```python
from build123d import *

# Parameters (mm, degrees)
BOSS_EXTRUDE1_DEPTH   = 3
BOSS_EXTRUDE2_DEPTH   = 3.5
BOSS_EXTRUDE3_DEPTH   = 3.7
SKETCH4_R             = 2.88
BOSS_EXTRUDE4_DEPTH   = 12
SKETCH9_W             = 6.5
SKETCH9_H             = 0.7
CUT_EXTRUDE2_DEPTH    = 23
F_2_5MM_DOWEL_HOLE1_D = 2.5
SKETCH8_R             = 1.6
CUT_EXTRUDE1_DEPTH    = 38.747052924
FILLET1_R             = 1
FILLET2_R             = 1
FILLET3_R             = 0.5


with BuildPart() as part:
    # Sketch1 → Boss-Extrude1 (new body)
    with BuildSketch(Plane(origin=(0, 0, 0), x_dir=(1, 0, 0), z_dir=(0, 1, 0))):
        with BuildLine():
            Line((0, 13), (16, 13))
            Line((16, 13), (16, 7))
            Line((16, 7), (0, 7))
            ThreePointArc((0, 7), (-7, 0), (0, -7))
            Line((0, -7), (16, -7))
            Line((16, -7), (16, -13))
            Line((16, -13), (0, -13))
            ThreePointArc((0, -13), (-13, 0), (0, 13))
        make_face()
    extrude(amount=BOSS_EXTRUDE1_DEPTH)

    # Sketch2 → Boss-Extrude2 (add)
    with BuildSketch(Plane(origin=(0, 3, 0), x_dir=(1, 0, 0), z_dir=(0, 1, 0))):
        with BuildLine():
            Line((0, 13), (16, 13))
            Line((16, 13), (16, 10))
            Line((16, 10), (0, 10))
            ThreePointArc((0, 10), (-10, 0), (0, -10))
            Line((0, -10), (16, -10))
            Line((16, -10), (16, -13))
            Line((16, -13), (0, -13))
            ThreePointArc((0, -13), (-13, 0), (0, 13))
        make_face()
    extrude(amount=BOSS_EXTRUDE2_DEPTH)

    # Sketch3 → Boss-Extrude3 (add)
    with BuildSketch(Plane(origin=(0, 6.5, 0), x_dir=(1, 0, 0), z_dir=(0, 1, 0))):
        with BuildLine():
            Line((16, 13), (0, 13))
            ThreePointArc((0, 13), (-13, 0), (0, -13))
            Line((0, -13), (16, -13))
            Line((16, -13), (16, -7))
            Line((16, -7), (16, 7))
            Line((16, 7), (16, 13))
        make_face()
    extrude(amount=BOSS_EXTRUDE3_DEPTH)

    # Sketch4 → Boss-Extrude4 (add)
    with BuildSketch(Plane(origin=(0, 10.2, 0), x_dir=(1, 0, 0), z_dir=(0, 1, 0))):
        with Locations(Location((0, 0, 0), (0, 0, 270))):
            Circle(SKETCH4_R)
    extrude(amount=BOSS_EXTRUDE4_DEPTH)

    # Sketch9 → Cut-Extrude2 (cut)
    with BuildSketch(Plane(origin=(16, 0, 0), x_dir=(0, 0, -1), z_dir=(1, 0, 0))):
        with Locations((0, 6.85)):
            Rectangle(SKETCH9_W, SKETCH9_H)
    extrude(amount=-CUT_EXTRUDE2_DEPTH, mode=Mode.SUBTRACT)

    # Ø2.5mm Dowel Hole1 (through all)
    with Locations(Plane(origin=(-0.002429038, 18.104937254, 2.879998976), x_dir=(0.999999644325, 0, 0.000843415861), z_dir=(-0.000843415861, 0, 0.999999644325))):
        with Locations((0, 0)):
            Hole(F_2_5MM_DOWEL_HOLE1_D / 2)

    # Sketch8 → Cut-Extrude1 (cut, through all)
    with BuildSketch(Plane.XY.offset(13)):
        with Locations((12.5, 5.1)):
            Circle(SKETCH8_R)
    extrude(amount=-CUT_EXTRUDE1_DEPTH, mode=Mode.SUBTRACT)

    # Fillet1
    fillet1_edges = [part.edges().sort_by_distance(p)[0] for p in [
        (8, 0, -13),
        (8, 0, -7),
        (-7, 0, 0),
        (16, 5.1, 13),
        (16, 5.1, -13),
        (-13, 10.2, 0),
        (8, 10.2, 13),
        (8, 10.2, -13),
        (8, 0, 7),
        (8, 0, 13),
        (-13, 0, 0),
    ]]
    fillet(fillet1_edges, radius=FILLET1_R)

    # Fillet2
    fillet2_edges = [part.edges().sort_by_distance(p)[0] for p in [
        (0, 10.2, -2.88),
    ]]
    fillet(fillet2_edges, radius=FILLET2_R)

    # Fillet3
    fillet3_edges = [part.edges().sort_by_distance(p)[0] for p in [
        (0, 22.2, -2.88),
    ]]
    fillet(fillet3_edges, radius=FILLET3_R)


solid = part.part
```
The model under review builds one solid part; all positions refer to its coordinate system, in mm. A direction names the side the tool comes from. Give positions to 0.01 mm unless a question says otherwise; leave off trailing zeros. Write each loop counter-clockwise with the first axis right and the second up, starting at its lowest first coordinate (ties: lowest second). Pieces come first, ordered by that corner, then holes. Notation, with made-up numbers: M 70,-17 L 119,-17 A25 ccw 119,4 Z; hole C 49.5,63 d9. An arc over 180 degrees is marked long. Answer in a Markdown table with one row per item.
Item 1: Add section A-A on y = 5.1. Give the boundary of the cut face in (x, z), plus the area to 3 significant figures.
Check sheet entries:
| item | result |
|---|---|
| outline | M 0,-13 L 10.9,-13 L 10.9,-10 L 0,-10 A10 cw 0,10 L 10.9,10 L 10.9,13 L 0,13 A13 ccw Z; M 14.1,-13 L 15,-13 A1 ccw 16,-12 L 16,-10 L 14.1,-10 Z; M 14.1,10 L 16,10 L 16,12 A1 ccw 15,13 L 14.1,13 Z |
| area | 185 mm2 |
Item 2: For P1, Ø12, axis at x = 3.5, y = 18, coming from the +Z side; P2, Ø0.8, axis at x = 14.5, z = 5.5, coming from the -Y side; P3, Ø3, axis at x = 8, z = -0.5, coming from the -Y side, all flat-tipped, find the tip position at first contact; note any pin that passes through.
Check sheet entries:
| item | result |
|---|---|
| P1 | z = 2.88 |
| P2 | y = 6.5 |
| P3 | y = 7.2 |
Item 3: Add section D-D on y = 14.25. Give the boundary of the cut face in (x, z).
Check sheet entries:
| item | result |
|---|---|
| outline | C 0,0 d5.76 |
Item 4: Tool access review of faces 1 (the face through (-10, 5, 0)), 2 (the face through (8.112, 0.285, 7.301)), 3 (the face through (-13, 5, 0)): name each direction out of +Z, -Z, +X, -X, +Y, -Y from which nothing blocks a thin tool from reaching the whole face with its end or side.
Check sheet entries:
| item | result |
|---|---|
| face 1 | +X |
| face 2 | +X, -Y |
| face 3 | -X, +Y, -Y |
Item 5: For line 1 along Z through (x, y) = (3.75, 3.75); line 2 along Y through (x, z) = (12.5, -9); line 3 along Y through (x, z) = (12.5, 5.75), list the stretches that pass through material, from the lowest coordinate up.
Check sheet entries:
| item | result |
|---|---|
| line 1 | -13 to -10, 10 to 13 |
| line 2 | 0 to 3, 6.7 to 10.2 |
| line 3 | 6.7 to 10.2 |
Item 6: Draft analysis for pull direction Z (two halves, no side actions). For faces 4 (the face through (15.715, 5.029, 12.699)), 5 (the face through (-1.752, 16.376, -2.285)), 6 (the face through (8, 2, 7)), 7 (the face through (2.2, 0, -8.2)), state which applies: +Z half, -Z half, draft (parallel to the pull), parting line (faces both ways), or undercut.
Check sheet entries:
| item | result |
|---|---|
| face 4 | +Z half |
| face 5 | parting line |
| face 6 | undercut |
| face 7 | draft |
Item 7: Add section B-B on x = 12.5. Give the boundary of the cut face in (y, z), plus the area to 3 significant figures.
Check sheet entries:
| item | result |
|---|---|
| outline | M 0,-12 A1 ccw 1,-13 L 3.5,-13 L 3.5,-10 L 3,-10 L 3,-7 L 1,-7 A1 ccw 0,-8 Z; M 0,8 A1 ccw 1,7 L 3,7 L 3,10 L 3.5,10 L 3.5,13 L 1,13 A1 ccw 0,12 Z; M 6.7,-13 L 9.2,-13 A1 ccw 10.2,-12 L 10.2,12 A1 ccw 9.2,13 L 6.7,13 L 6.7,3.25 L 7.2,3.25 L 7.2,-3.25 L 6.7,-3.25 Z |
| area | 125 mm2 |
Item 8: Add section C-C on y = 8. Give the boundary of the cut face in (x, z), plus the area to 3 significant figures.
Check sheet entries:
| item | result |
|---|---|
| outline | M 0,-13 L 15,-13 A1 ccw 16,-12 L 16,12 A1 ccw 15,13 L 0,13 A13 ccw Z |
| area | 681 mm2 |
